Autodesk Inventor part; units mm, degrees
ref_plane "YZ Plane" through (0, 0, 0) normal (1, 0, 0) x (0, 1, 0)
ref_plane "XZ Plane" through (0, 0, 0) normal (0, 1, 0) x (-1, 0, 0)
ref_plane "XY Plane" through (0, 0, 0) normal (0, 0, 1) x (1, 0, 0)
sketch "スケッチ1" plane through (0, 0, 0) normal (0, 0, 1) x (1, 0, 0)
  line L0 (0, 0) -> (-2.7189, -1.2679) construction
  line L1 (0, 0) -> (0, -26) construction
  arc A0 (8.8407, -4.1114) -> (-9.5086, -2.1563) centre (0, 0) ccw
  arc A1 (-3.901, -26.8846) -> (4, -26) centre (0, -26) ccw
  arc A2 (8.8407, -4.1114) -> (4, -26) centre (55.9076, -26) ccw
  line L2 (-9.5086, -2.1563) -> (-3.901, -26.8846)
  line L3 (0, -26) -> (4, -26) construction
  circle A3 centre (0, 0) radius 8 construction
  point P0 (8, 0)
  point P1 (5.6569, 5.6569)
  point P2 (0, 8)
  point P3 (-5.6569, 5.6569)
  point P4 (-8, 0)
  point P5 (-5.6569, -5.6569)
  point P6 (0, -8)
  point P7 (5.6569, -5.6569)
  point P8 (0, -26)
  dimension "d38" = 16
  dimension "d2" = 3
  dimension "d4" = 26
  dimension "d6" = 9.75
  dimension "d7" = 4
  dimension "d11" = 360
  dimension "d37" = 65
extrude "押し出し1" add sketch "スケッチ1" along normal blind 3
sketch "スケッチ5" plane through (0, 0, 3) normal (0, 0, 1) x (1, 0, 0)
  circle A0 centre (0, 0) radius 6
  arc A1 (8.8407, -4.1114) -> (-9.5086, -2.1563) centre (0, 0) ccw construction
  dimension "d41" = 12
extrude "押し出し4" add sketch "スケッチ5" along normal blind 2.5
hole "穴1" at (8, 0, 0) at (5.6569, 5.6569, 0) at (0, 8, 0) at (-5.6569, 5.6569, 0) at (-8, 0, 0) at (-5.6569, -5.6569, 0) at (0, -8, 0) at (5.6569, -5.6569, 0) direction (0, 0, 1) diameter 2 end through all
hole "穴2" at (0, -26, 0) direction (0, 0, 1) diameter 3 end through all
sketch "スケッチ2" plane through (0, 0, 0) normal (0, 0, -1) x (-1, 0, 0)
  circle A0 centre (0, 0) radius 4
  dimension "d30" = 8
extrude "押し出し2" cut sketch "スケッチ2" against normal blind 2
sketch "スケッチ3" plane through (0, 0, 5.5) normal (0, 0, 1) x (1, 0, 0)
  circle A0 centre (-2.7189, -1.2679) radius 2
  point P0 (0, 0)
  dimension "d33" = 4
extrude "押し出し3" add sketch "スケッチ3" along normal blind 3.2
chamfer "面取り1" distance 0.5 angle 45 5 edges at (-6, 0, 5.5) (1.033, 9.6951, 3) (-6.7048, -14.5204, 3) (0.4451, -29.9752, 3) (5.2246, -14.7913, 3)
properties part number "COXA_ROLL_SERVO-OUTPUT"
CAD build for the part. Positions are in the model's coordinates, mm. A direction names the side the tool comes from. Coordinates: 2 decimals unless noted, no trailing zeros. Write each loop counter-clockwise with the first axis right and the second up, starting at its lowest first coordinate (ties: lowest second). Pieces come first, ordered by that corner, then holes. Notation, with made-up numbers: M 83,9 L 110,9 A19 cw 110,14 Z; hole C -29.5,19 d9. An arc over 180 degrees is marked long. Return JSON: item names as keys, results as strings.
Item 1: Slice it at C-C, the plane z = 7.5. Write the cut outline in (x, y), and give its area (3 significant figures).
Findings below:
{"outline": "C -2.72,-1.27 d4", "area": "12.6 mm2"}
Item 2: Probe line 1 (Y direction, x = 0, z = 2.1); line 2 (Y direction, x = 0, z = 0.55); line 3 (Z direction, x = 1.5, y = -8). List the from-to ranges inside material, lowest first. Write a range as from..to.
Findings below:
{"line 1": "y = -30..-27.5, -24.5..-9, -7..7, 9..9.75", "line 2": "y = -30..-27.5, -24.5..-9, -7..-4, 4..7, 9..9.75", "line 3": "z = 0..3"}
Item 3: Slice it at A-A, the plane z = 0.5. State how many separate pieces and enclosed holes the cut face has, and give its area (3 significant figures).
Findings below:
{"separate pieces": "1", "enclosed holes": "10", "area": "436 mm2"}
Item 4: Which spindle directions (+Z, -Z, +X, -X, +Y, -Y) get a long thin tool onto all of the face, cutting with end or side? Do faces 4 (the cylindrical face through (-6, 0, 4)), 5 (the cylindrical face through (0.867, -3.905, 0.986)), 6 (the cylindrical face through (-0.07, -27.5, 1.52)). Say none if no direction does.
Findings below:
{"face 4": "+Z", "face 5": "-Z", "face 6": "+Z, -Z"}
Item 5: Two-plate mould, pull along Y, no slides. Class faces 1 (the flat face through (-3, -1, 8.7)), 2 (the flat face through (-6.42, -14.64, 2.75)), 3 (the cylindrical face through (-6.333, -6.394, 1.521)): +Y half, -Y half, draft (parallel to the pull), parting line (faces both ways), or undercut.
Findings below:
{"face 1": "draft", "face 2": "-Y half", "face 3": "undercut"}
Item 6: Drop flat-ended pins along their axis: pin 1 Ø2.5 at (x, y) = (-8, 0) entering from +Z; pin 2 Ø3 at (x, z) = (1, 5.5) entering from +Y; pin 3 Ø3 at (x, y) = (6, -18) entering from +Z. Give the stop position or say it passes through.
Findings below:
{"pin 1": "stops at z = 3", "pin 2": "stops at y = 6", "pin 3": "stops at z = 2.64"}
